Geometry check sheet. Reference: the model listing, model coordinates, mm. Face numbers are marked on the shaded views. A direction names the side the tool comes from. Round coordinates to 2 decimals unless told otherwise and drop trailing zeros. Order: outer loops, then holes, each group sorted by start corner. A loop starts at its lowest first (then second) coordinate and runs counter-clockwise, first axis right, second up.
(1) Release check for a two-part mould opening along X. For the marked faces 1, 2, 3 and 4 record: +X half, -X half, draft (parallel to the pull), parting line (faces both ways), or undercut.
(2) Set-up check for the marked faces 5, 6, 7 and 8: record each of +Z, -Z, +X, -X, +Y, -Y from which the full face is reachable in a straight line by a thin tool's end or side.
(3) Material ranges on line 1 along Y through (x, z) = (0, 4); line 2 along X through (y, z) = (-4.5, 0.8); line 3 along Y through (x, z) = (-4.75, 4.9), recorded low to high.
(4) Sectioned sample at A-A (y = 0). Record the boundary of the cut face in (x, z), plus the area to 3 significant figures.
(5) Sectioned sample at B-B (x = 0). Record the boundary of the cut face in (y, z), plus the area to 3 significant figures.
(6) Go/stop test with flat-tipped pins: pin 1 (1.5 mm diameter, centred on x = -4, y = -1, fed in from +Z); pin 2 (2 mm diameter, centred on y = -3, z = 3, fed in from +X); pin 3 (2.5 mm diameter, centred on x = 0, y = 0, fed in from -Z). Record where each tip stops, or that it passes through.
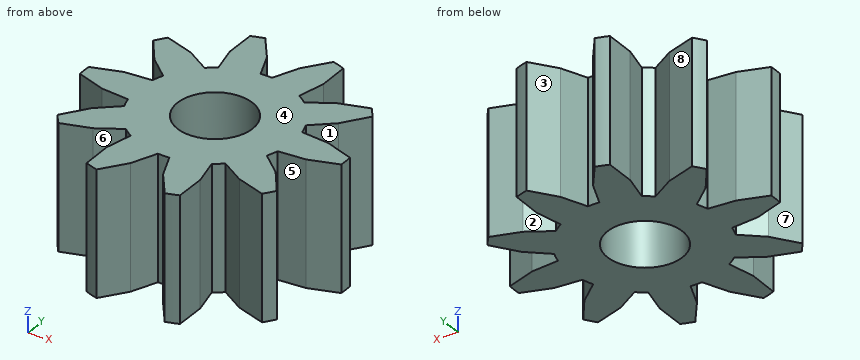
from build123d import *

# Parameters (mm, degrees)
SKETCH1_R           = 5.75
BOSS_EXTRUDE1_DEPTH = 5.5
SKETCH2_R           = 1.65
CUT_EXTRUDE1_DEPTH  = 5.5
CUT_EXTRUDE3_START  = -5.5
CUT_EXTRUDE3_DEPTH  = 5.5
CIRPATTERN2_COUNT   = 10


with BuildPart() as part:
    # Sketch1 → Boss-Extrude1 (new body)
    with BuildSketch(Plane.XY):
        Circle(SKETCH1_R)
    extrude(amount=BOSS_EXTRUDE1_DEPTH)

    # Sketch2 → Cut-Extrude1 (cut)
    with BuildSketch(Plane.XY.offset(5.5)):
        Circle(SKETCH2_R)
    extrude(amount=-CUT_EXTRUDE1_DEPTH, mode=Mode.SUBTRACT)

    # Sketch5 → Cut-Extrude3 (cut)
    with BuildSketch(Plane.XY.offset(5.5).offset(CUT_EXTRUDE3_START)):
        with BuildLine():
            Line((-0.25, 3.376770386), (-0.711246658, 4.479961461))
            Line((-0.711246658, 4.479961461), (-1.5, 5.550900828))
            ThreePointArc((-1.5, 5.550900828), (0, 5.75), (1.5, 5.550900828))
            Line((1.5, 5.550900828), (0.715828266, 4.487930272))
            Line((0.715828266, 4.487930272), (0.25, 3.376770386))
            ThreePointArc((0.25, 3.376770386), (0, 3.386012144), (-0.25, 3.376770386))
        make_face()
    cut_extrude3 = extrude(amount=CUT_EXTRUDE3_DEPTH, mode=Mode.SUBTRACT)

    # CirPattern2: Cut-Extrude3 ×10 about axis
    cirpattern2_axis = Axis((0, 0, 0), (0, 0, 1))
    for i in range(1, CIRPATTERN2_COUNT):
        add(cut_extrude3.rotate(cirpattern2_axis, i * 360 / CIRPATTERN2_COUNT), mode=Mode.SUBTRACT)


solid = part.part
Answer below:
1. face 1: +X half
1. face 2: undercut
1. face 3: undercut
1. face 4: draft
2. face 5: +Z, -Z, +X
2. face 6: +Z, -Z, -Y
2. face 7: +Z, -Z, -X
2. face 8: +Z, -Z, +Y
3. line 1: y = -3.39 to -1.65, 1.65 to 3.39
3. line 2: x = -2.05 to -0.72, 0.73 to 2.06
3. line 3: y = -3.24 to -3.05, -0.62 to 0.62, 3.05 to 3.24
4. outline: (-5.75, 0) - (-1.65, 0) - (-1.65, 5.5) - (-5.75, 5.5) - close; (1.65, 0) - (5.75, 0) - (5.75, 5.5) - (1.65, 5.5) - close
4. area: 45.1 mm2
5. outline: (-3.39, 0) - (-1.65, 0) - (-1.65, 5.5) - (-3.39, 5.5) - close; (1.65, 0) - (3.39, 0) - (3.39, 5.5) - (1.65, 5.5) - close
5. area: 19.1 mm2
6. pin 1: stops at z = 5.5
6. pin 2: stops at x = 4.82
6. pin 3: passes through
